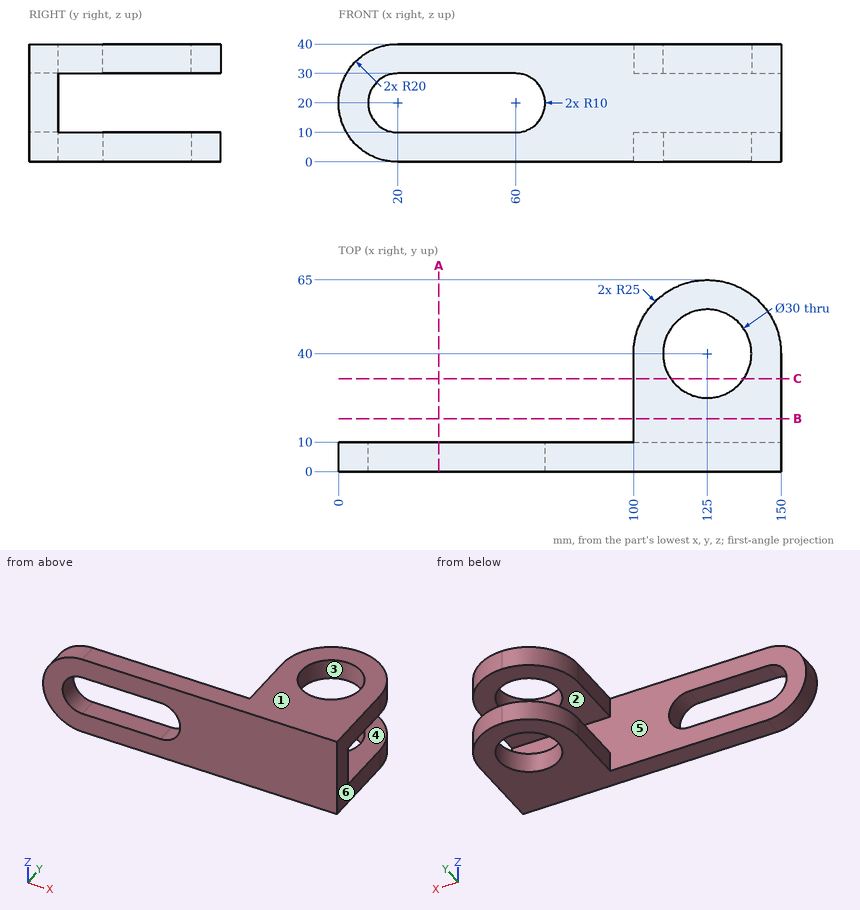
The figure shows three views and two pictorial views of one solid part (mm, origin at its lowest corner). Answer the questions. A direction names the side the tool comes from. Coordinates: 2 decimals unless noted, no trailing zeros. Loops run counter-clockwise (first coordinate to the right, second up) from the corner with the lowest first, then second, coordinate; pieces in that order, holes last.
(1) The part is cut by section B-B (y = 18). Determine the outline of the cut face in (x, z).
Solution:
outline: (100, 0) - (150, 0) - (150, 10) - (100, 10) - close; (100, 30) - (150, 30) - (150, 40) - (100, 40) - close
(2) The part is cut by section A-A (x = 34). Determine the outline of the cut face in (y, z).
Solution:
outline: (0, 0) - (10, 0) - (10, 10) - (0, 10) - close; (0, 30) - (10, 30) - (10, 40) - (0, 40) - close
(3) Consider line 1 along Y through (x, z) = (125, 6.25); line 2 along Z through (x, y) = (124, 56); line 3 along X through (y, z) = (29, 2.5). Determine where each line is inside the solid, lowest interval first.
Solution:
line 1: y = 0 to 25, 55 to 65
line 2: z = 0 to 10, 30 to 40
line 3: x = 100 to 114.8, 135.2 to 150
(4) A tool of negligible diameter and unlimited length cuts with its end or side. For the marked faces 4, 5 and 6, from which of +Z, -Z, +X, -X, +Y, -Y can it reach the whole face along a straight path? Write none if from no direction.
Solution:
face 4: +X, -X, +Y
face 5: -X, +Y
face 6: +Z, -Z, +X, +Y, -Y
(5) The part is cut by section C-C (y = 31.5). Determine the outline of the cut face in (x, z), and give its area (3 significant figures).
Solution:
outline: (100, 0) - (112.64, 0) - (112.64, 10) - (100, 10) - close; (100, 30) - (112.64, 30) - (112.64, 40) - (100, 40) - close; (137.36, 0) - (150, 0) - (150, 10) - (137.36, 10) - close; (137.36, 30) - (150, 30) - (150, 40) - (137.36, 40) - close
area: 506 mm2
(6) Flat-ended cylindrical pins translate along their axes: pin 1 Ø4 at (y, z) = (58.5, 10) entering from +X; pin 2 Ø1 at (x, y) = (98, 23) entering from -Z; pin 3 Ø5 at (y, z) = (27, 8) entering from -X; pin 4 Ø3 at (x, z) = (41, 31) entering from +Y. Find the tip coordinate at first contact, or state that the pin passes through.
Solution:
pin 1: stops at x = 143.78
pin 2: passes through
pin 3: stops at x = 100
pin 4: stops at y = 10
(7) The mould has two halves that part along Z. Classify the marked faces 1, 2 and 3: released by +Z, released by -Z, zero draft, split by the parting line, or undercut.
Solution:
face 1: released by +Z
face 2: undercut
face 3: zero draft
